Autodesk Inventor part; units mm, degrees
ref_plane "YZ Plane" through (0, 0, 0) normal (1, 0, 0) x (0, 1, 0)
ref_plane "XZ Plane" through (0, 0, 0) normal (0, 1, 0) x (-1, 0, 0)
ref_plane "XY Plane" through (0, 0, 0) normal (0, 0, 1) x (1, 0, 0)
sketch "Sketch1" plane through (0, 0, 0) normal (0, 1, 0) x (-1, 0, 0)
  line L0 (0, 0) -> (-19.05, 0)
  line L1 (-19.05, 0) -> (-19.05, 133.35)
  line L2 (-19.05, 133.35) -> (0, 133.35)
  line L3 (0, 133.35) -> (0, 0)
  dimension "d0" = 19.05
  dimension "d1" = 133.35
extrude "Board" add sketch "Sketch1" along normal blind 857.25
sketch "Sketch2" plane through (19.05, 0, 133.35) normal (1, 0, 0) x (0, 0, -1)
  line L0 (0, 425.45) -> (133.35, 425.45)
  line L1 (133.35, 425.45) -> (133.35, 406.4)
  line L2 (133.35, 406.4) -> (0, 406.4)
  line L3 (0, 406.4) -> (0, 425.45)
  line L4 (0, 0) -> (133.35, 0)
  line L5 (0, 0) -> (0, 857.25)
  line L6 (133.35, 0) -> (133.35, 857.25)
  dimension "d4" = 19.05
  dimension "d5" = 406.4
extrude "Shelf Notch" cut sketch "Sketch2" against normal blind 9.525 contours L0 L1 L2 L3
sketch "Sketch3" plane through (0, 0, 133.35) normal (0, 0, 1) x (1, 0, 0)
  line L0 (0, 857.25) -> (19.05, 857.25)
  line L1 (0, 857.25) -> (9.525, 857.25)
  line L2 (9.525, 857.25) -> (9.525, 847.725)
  line L3 (9.525, 847.725) -> (0, 847.725)
  line L4 (0, 847.725) -> (0, 857.25)
  line L5 (0, 0) -> (9.525, 0)
  line L6 (9.525, 0) -> (9.525, 9.525)
  line L7 (9.525, 9.525) -> (0, 9.525)
  line L8 (0, 9.525) -> (0, 0)
  dimension "d8" = 9.525
  dimension "d9" = 9.525
  dimension "d14" = 9.525
  dimension "d15" = 9.525
extrude "Top and Bottom Dados" cut sketch "Sketch3" against normal blind 133.35
sketch "Sketch5" plane through (0, 9.525, 0) normal (-1, 0, 0) x (0, 0, 1)
  line L0 (122.2375, 647.7) -> (133.35, 647.7)
  line L1 (133.35, 647.7) -> (133.35, 609.6)
  line L2 (133.35, 609.6) -> (122.2375, 609.6)
  line L3 (119.0625, 612.775) -> (119.0625, 644.525)
  line L4 (133.35, 838.2) -> (0, 838.2)
  line L5 (133.35, 0) -> (133.35, 838.2)
  line L6 (122.2375, 228.6) -> (133.35, 228.6)
  line L7 (133.35, 228.6) -> (133.35, 190.5)
  line L8 (133.35, 190.5) -> (122.2375, 190.5)
  line L9 (119.0625, 193.675) -> (119.0625, 225.425)
  line L10 (0, 0) -> (133.35, 0)
  arc A0 (122.2375, 647.7) -> (119.0625, 644.525) centre (122.2375, 644.525) ccw
  arc A1 (119.0625, 612.775) -> (122.2375, 609.6) centre (122.2375, 612.775) ccw
  arc A2 (122.2375, 228.6) -> (119.0625, 225.425) centre (122.2375, 225.425) ccw
  arc A3 (119.0625, 193.675) -> (122.2375, 190.5) centre (122.2375, 193.675) ccw
  point P0 (0, -9.525)
  point P1 (119.0625, 609.6)
  point P2 (119.0625, 190.5)
  dimension "d16" = 14.2875
  dimension "d17" = 38.1
  dimension "d18" = 838.2
  dimension "d19" = 190.5
  dimension "d20" = 38.1
  dimension "d21" = 14.2875
  dimension "d22" = 381
  dimension "d24" = 3.175
extrude "Hinge" cut sketch "Sketch5" against normal blind 3.175
equation "\"d12\" = d1"
equation "\"d19\" = 0.25 * d18 - 0.5 * d17"
equation "\"d20\" = d17"
equation "\"d22\" = 2 * d19"
properties part number "Door Side"
Geometry: final body of the model. Coordinates: model frame, mm. A direction names the side the tool comes from. Give positions to 0.01 mm unless a question says otherwise; leave off trailing zeros. Loops run counter-clockwise (first coordinate to the right, second up) from the corner with the lowest first, then second, coordinate; pieces in that order, holes last. Notation, with made-up numbers: (-30, 30) -> (-16, 30) arc R35 cw to (-16, 63) -> close; hole circle Ø11 at (14.5, 22). An arc over 180 degrees is marked (long way). Use CSV: the item, a comma, the result in double quotes.
(1) Access query for faces 4 (the face through (3.175, 219, 126)), 5 (the face through (9, 423, 0)). Directions: +Z, -Z, +X, -X, +Y, -Y. A direction counts if a zero-diameter tool reaches every point of the face in a straight line with its end or side. Return the directions, or none.
From the geometry:
face 4,"+Z, -X"
face 5,"-Z, +X, -X, +Y, -Y"
(2) Pull-direction query (Y, two-part tool) for faces 1 (the face through (9.525, 416, 68)), 2 (the face through (3.175, 638, 126)), 3 (the face through (19.05, 638, 66)); classes: released by +Y, released by -Y, zero draft, split by the parting line, or undercut.
From the geometry:
face 1,"undercut"
face 2,"undercut"
face 3,"zero draft"
(3) Ray query, line 1 along Y through (x, z) = (18.25, 81.5); line 2 along Y through (x, z) = (1.25, 68) (3 decimals); line 3 along X through (y, z) = (655, 125) (3 decimals). Return the intervals inside material, ascending. Write a range as [from, to].
From the geometry:
line 1,"[0, 406.4], [425.45, 857.25]"
line 2,"[9.525, 847.725]"
line 3,"[3.175, 19.05]"
(4) First-contact query: P1, Ø7.5, axis at x = 5, z = 47, coming from the -Y side (3 decimals); P2, Ø5, axis at y = 851.5, z = 100, coming from the -X side (3 decimals); P3, Ø4.5, axis at y = 635.5, z = 125, coming from the -X side (3 decimals); P4, Ø10.5, axis at x = 14.5, z = 52.5, coming from the -Y side. Flat tips, straight axial feed; report the tip coordinate or a pass-through.
From the geometry:
P1,"y = 9.525"
P2,"x = 9.525"
P3,"x = 3.175"
P4,"y = 0"
(5) Cut plane B-B (z = 69.5). Output: boundary loops of the cut face in (x, y) (3 decimals), plus the area to 3 significant figures.
From the geometry:
outline,"(0, 9.525) -> (9.525, 9.525) -> (9.525, 0) -> (19.05, 0) -> (19.05, 406.4) -> (9.525, 406.4) -> (9.525, 425.45) -> (19.05, 425.45) -> (19.05, 857.25) -> (9.525, 857.25) -> (9.525, 847.725) -> (0, 847.725) -> close"
area,"16,000 mm^2"
(6) Cut plane A-A (x = 14.75). Output: boundary loops of the cut face in (y, z).
From the geometry:
outline,"(0, 0) -> (406.4, 0) -> (406.4, 133.35) -> (0, 133.35) -> close; (425.45, 0) -> (857.25, 0) -> (857.25, 133.35) -> (425.45, 133.35) -> close"
